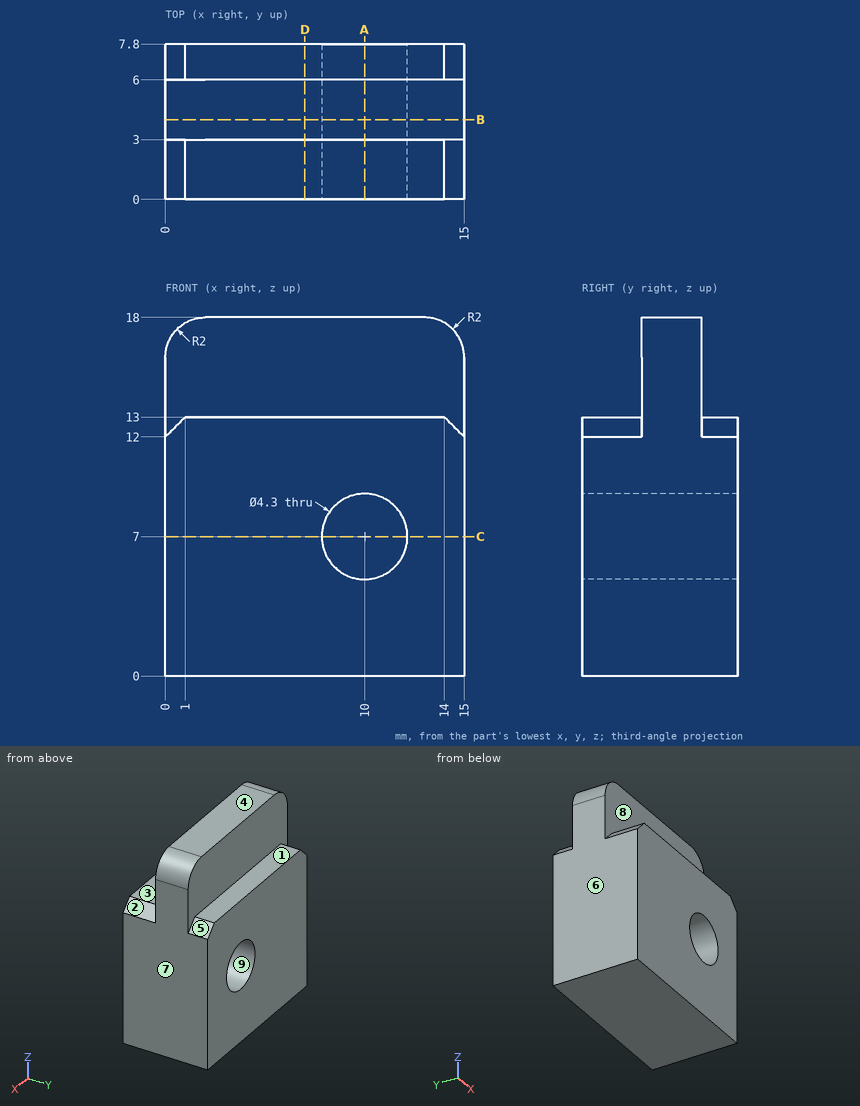
The figure shows three views and two pictorial views of one solid part (mm, origin at its lowest corner). Answer the questions. A direction names the side the tool comes from. Round coordinates to 2 decimals unless told otherwise and drop trailing zeros. Order: outer loops, then holes, each group sorted by start corner. A loop starts at its lowest first (then second) coordinate and runs counter-clockwise, first axis right, second up.
Q1. A cutting plane is placed at C-C, the plane z = 7. Determine the outline of the cut face in (x, y).
Solution:
outline: (0, 0) - (7.85, 0) - (7.85, 7.8) - (0, 7.8) - close; (12.15, 0) - (15, 0) - (15, 7.8) - (12.15, 7.8) - close
Q2. A cutting plane is placed at D-D, the plane x = 7. Determine the outline of the cut face in (y, z), then the cut area to 3 significant figures.
Solution:
outline: (0, 0) - (7.8, 0) - (7.8, 13) - (6, 13) - (6, 18) - (3, 18) - (3, 13) - (0, 13) - close
area: 116 mm2
Q3. Find the intervals of material crossed by line 1 along Z through (x, y) = (10, 5); line 2 along Z through (x, y) = (10, 6.25); line 3 along Z through (x, y) = (13.25, 7.5), in increasing order.
Solution:
line 1: z = 0 to 4.85, 9.15 to 18
line 2: z = 0 to 4.85, 9.15 to 13
line 3: z = 0 to 13
Q4. A cutting plane is placed at B-B, the plane y = 4. Determine the outline of the cut face in (x, z), then the cut area to 3 significant figures.
Solution:
outline: (0, 0) - (15, 0) - (15, 16) arc R2 ccw to (13, 18) - (2, 18) arc R2 ccw to (0, 16) - close; hole circle Ø4.3 at (10, 7)
area: 254 mm2
Q5. The mould has two halves that part along X. Classify the marked faces 6, 7, 8 and 9: pulls with the +X half, pulls with the -X half, needs draft (parallel to the pull), parting line crosses it, or undercut.
Solution:
face 6: pulls with the -X half
face 7: pulls with the +X half
face 8: needs draft
face 9: undercut
Q6. Given pin 1 Ø5 at (x, z) = (4, 16) entering from -Y; pin 2 Ø1.5 at (x, y) = (6, 1) entering from +Z, each flat-ended and moving along its own axis, determine where each tip first touches the part or whether it passes through.
Solution:
pin 1: stops at y = 3
pin 2: stops at z = 13
Q7. A tool of negligible diameter and unlimited length cuts with its end or side. For the marked faces 1, 2, 3, 4 and 5, from which of +Z, -Z, +X, -X, +Y, -Y can it reach the whole face along a straight path? Write none if from no direction.
Solution:
face 1: +Z, +X, -X, +Y
face 2: +Z, +X, -Y
face 3: +Z, +X, -X, -Y
face 4: +Z, +X, -X, +Y, -Y
face 5: +Z, +X, +Y
Q8. A cutting plane is placed at A-A, the plane x = 10. Determine the outline of the cut face in (y, z), then the cut area to 3 significant figures.
Solution:
outline: (0, 0) - (7.8, 0) - (7.8, 4.85) - (0, 4.85) - close; (0, 9.15) - (7.8, 9.15) - (7.8, 13) - (6, 13) - (6, 18) - (3, 18) - (3, 13) - (0, 13) - close
area: 82.9 mm2
